Input: part model. Units: mm. Frame: model coordinates. Face numbers are marked on the shaded views. Give positions to 0.01 mm unless a question says otherwise; leave off trailing zeros. Write each loop counter-clockwise with the first axis right and the second up, starting at its lowest first coordinate (ties: lowest second). Pieces come first, ordered by that corner, then holes. Notation, with made-up numbers: M -24.75,75.5 L 20.25,75.5 A16 cw 20.25,86.5 Z; hole C 2,-3 d7. An arc over 180 degrees is marked long. Use CSV: the item, a comma, the result in double quotes. Start each with the question number.
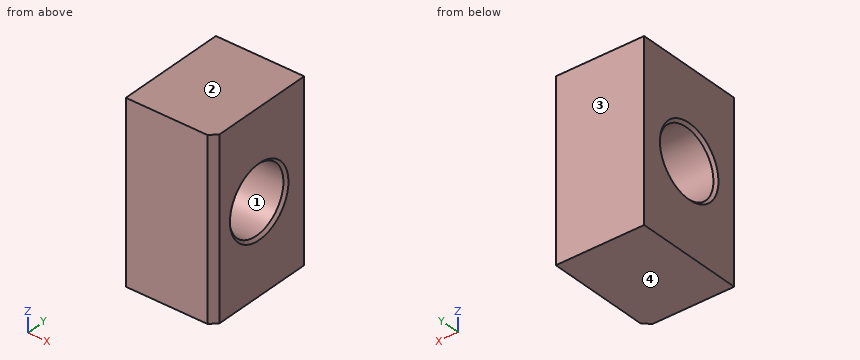
from build123d import *

# Parameters (mm, degrees)
SKETCH_1_W      = 4
SKETCH_1_H      = 5
EXTRUDE_1_DEPTH = 8
CHAMFER_1_SIZE  = 0.3


with BuildPart() as part:
    # Эскиз1 → Бобышка-Вытянуть1 (new body)
    with BuildSketch(Plane.XY):
        Rectangle(SKETCH_1_W, SKETCH_1_H)
    extrude(amount=EXTRUDE_1_DEPTH)

    # Эскиз2 → Отверстие обработанное метчиком M31 (revolve, cut)
    with BuildSketch(Plane(origin=(-2, 0, 4), x_dir=(0, 0, 1), z_dir=(0, 1, 0))):
        Polygon((0, 0), (0, 4), (1.625, 4), (1.5, 3.875), (1.5, 0.125), (1.625, 0), align=None)
    revolve(axis=Axis((-8.35, 0, 4), (1, 0, 0)), mode=Mode.SUBTRACT)

    # Фаска1
    chamfer_1_edges = [part.edges().sort_by_distance(p)[0] for p in [
        (2, -2.5, 4),
    ]]
    chamfer(chamfer_1_edges, length=CHAMFER_1_SIZE)


solid = part.part
Q1. Material intervals for L1, parallel to Z at x = 0.9, y = 0; L2, parallel to Y at x = -1, z = 4; L3, parallel to Y at x = -1.15, z = 3.5, sorted ascending. Write a range as [from, to].
Q2. Pull-direction query (Z, two-part tool) for the marked faces 1, 2, 3 and 4; classes: released by +Z, released by -Z, zero draft, split by the parting line, or undercut.
Q3. Section B-B, the plane y = 0. Return the cut outline in (x, z) (3 decimals).
Q4. First-contact query: pin 1 Ø2.5 at (y, z) = (0, 4) entering from +X. Flat tip, straight axial feed; report the tip coordinate or a pass-through.
Q5. Section C-C, the plane x = 0.9. Return the cut outline in (y, z), and give its area (3 significant figures).
Q6. Section A-A, the plane z = 4. Return the cut outline in (x, y) (3 decimals).
Check result:
1,L1,"z = [0, 2.5], [5.5, 8]"
1,L2,"y = [-2.5, -1.5], [1.5, 2.5]"
1,L3,"y = [-2.5, -1.41], [1.41, 2.5]"
2,face 1,"undercut"
2,face 2,"released by +Z"
2,face 3,"zero draft"
2,face 4,"released by -Z"
3,outline,"M -2,0 L 2,0 L 2,2.375 L 1.875,2.5 L -1.875,2.5 L -2,2.375 Z; M -2,5.625 L -1.875,5.5 L 1.875,5.5 L 2,5.625 L 2,8 L -2,8 Z"
4,pin 1,"passes through"
5,outline,"M -2.5,0 L 2.5,0 L 2.5,8 L -2.5,8 Z; hole C 0,4 d3"
5,area,"32.9 mm²"
6,outline,"M -2,-2.5 L 1.7,-2.5 L 2,-2.2 L 2,-1.625 L 1.875,-1.5 L -1.875,-1.5 L -2,-1.625 Z; M -2,1.625 L -1.875,1.5 L 1.875,1.5 L 2,1.625 L 2,2.5 L -2,2.5 Z"
